```python
from build123d import *

# Parameters (mm, degrees)
SKETCH_1_W          = 80
SKETCH_1_H          = 50
EXTRUDE_1_DEPTH     = 100
SKETCH_3_W          = 66
SKETCH_3_H          = 44.469830213
CUT_EXTRUDE_1_DEPTH = 138.477270849
SKETCH_4_R          = 2.1
CUT_EXTRUDE_2_DEPTH = 138.477270849


with BuildPart() as part:
    # 草圖1 → 填料-伸長1 (new body)
    with BuildSketch(Plane(origin=(0, 0, 0), x_dir=(1, 0, 0), z_dir=(0, 1, 0))):
        with Locations((40, 25)):
            Rectangle(SKETCH_1_W, SKETCH_1_H)
    extrude(amount=EXTRUDE_1_DEPTH)

    # 草圖3 → 除料-伸長1 (cut, through all)
    with BuildSketch(Plane(origin=(0, 0, 0), x_dir=(1, 0, 0), z_dir=(0, 1, 0))):
        with Locations((40, 29.234915107)):
            Rectangle(SKETCH_3_W, SKETCH_3_H)
    extrude(amount=CUT_EXTRUDE_1_DEPTH, mode=Mode.SUBTRACT)

    # 草圖4 → 除料-伸長2 (cut, through all)
    with BuildSketch(Plane(origin=(0, 0, 0), x_dir=(1, 0, 0), z_dir=(0, 1, 0))):
        with Locations(Location((3.5, 3.5, 0), (0, 0, 270))):
            Circle(SKETCH_4_R)
        with Locations(Location((3.5, 43.5, 0), (0, 0, 270))):
            Circle(SKETCH_4_R)
        with Locations(Location((76.5, 43.4, 0), (0, 0, 270))):
            Circle(SKETCH_4_R)
        with Locations(Location((76.5, 3.5, 0), (0, 0, 270))):
            Circle(SKETCH_4_R)
    extrude(amount=CUT_EXTRUDE_2_DEPTH, mode=Mode.SUBTRACT)


solid = part.part
```
Verification items for the finished model (mm, model axes). A direction names the side the tool comes from. Give positions to 0.01 mm unless a question says otherwise; leave off trailing zeros. Order: outer loops, then holes, each group sorted by start corner. A loop starts at its lowest first (then second) coordinate and runs counter-clockwise, first axis right, second up. Notation, with made-up numbers: M -32,5 L 13,5 A16 cw 13,14 Z; hole C 11,20.5 d4. An arc over 180 degrees is marked long. Return JSON: item names as keys, results as strings. Group by question number.
1) Section check D-D on z = -3.5. Record the cut outline in (x, y), and give its area (3 significant figures).
2) Access from +Z, -Z, +X, -X, +Y, -Y to the whole of each face (thin tool, end or side, straight path). Record for faces 4 (the face through (7, 49, -28)), 5 (the face through (0, 49, -25)).
3) Section check B-B on x = 76.5. Record the cut outline in (y, z).
4) Mould release check, pull along Z, two halves, no side actions. Record for faces 1 (the face through (39.8, 0, -6.6)), 2 (the face through (39, 49, 0)), 3 (the face through (1.45, 49.3, -43.96)): pulls with the +Z half, pulls with the -Z half, needs draft (parallel to the pull), parting line crosses it, or undercut.
5) Scan lines: line 1 (X direction, y = 54.5, z = -43.5); line 2 (Z direction, x = 76.5, y = 68); line 3 (X direction, y = 69.5, z = -4). Record each from-to range of solid material in increasing order.
6) Section check C-C on y = 8. Record the cut outline in (x, z), and give its area (3 significant figures).
7) Go/stop test with a flat-tipped pin: pin 1 Ø4 at (x, y) = (47.5, 27.5) entering from -Z. Record where the tip stops, or that it passes through.
8) Section check A-A on z = -12. Record the cut outline in (x, y), and give its area (3 significant figures).
Answer block:
{
 "1": {"outline": "M 0,0 L 1.4,0 L 1.4,100 L 0,100 Z; M 5.6,0 L 74.4,0 L 74.4,100 L 5.6,100 Z; M 78.6,0 L 80,0 L 80,100 L 78.6,100 Z", "area": "7,160 mm^2"},
 "2": {"face 4": "-Z, +Y, -Y", "face 5": "+Z, -Z, -X, +Y, -Y"},
 "3": {"outline": "M 0,-50 L 100,-50 L 100,-45.5 L 0,-45.5 Z; M 0,-41.3 L 100,-41.3 L 100,-5.6 L 0,-5.6 Z; M 0,-1.4 L 100,-1.4 L 100,0 L 0,0 Z"},
 "4": {"face 1": "needs draft", "face 2": "pulls with the +Z half", "face 3": "undercut"},
 "5": {"line 1": "x = 0 to 1.4, 5.6 to 7, 73 to 74.4, 78.6 to 80", "line 2": "z = -50 to -45.5, -41.3 to -5.6, -1.4 to 0", "line 3": "x = 0 to 1.46, 5.54 to 74.46, 78.54 to 80"},
 "6": {"outline": "M 0,-50 L 7,-50 L 7,-7 L 73,-7 L 73,-50 L 80,-50 L 80,0 L 0,0 Z; hole C 3.5,-43.5 d4.2; hole C 3.5,-3.5 d4.2; hole C 76.5,-43.4 d4.2; hole C 76.5,-3.5 d4.2", "area": "1,110 mm^2"},
 "7": {"pin 1": "stops at z = -7"},
 "8": {"outline": "M 0,0 L 7,0 L 7,100 L 0,100 Z; M 73,0 L 80,0 L 80,100 L 73,100 Z", "area": "1,400 mm^2"}
}
